from build123d import *

# Parameters (mm, degrees)
BOSS_EXTRUDE1_DEPTH  = 30
SHELL1_T             = -2
BOSS_EXTRUDE8_START  = -28
SKETCH10_R           = 1.25
BOSS_EXTRUDE8_DEPTH  = 28
BOSS_EXTRUDE10_START = 10
SKETCH4_R            = 2.7
BOSS_EXTRUDE10_DEPTH = 2.7
LPATTERN1_COUNT      = 4
LPATTERN1_PITCH      = 25
SKETCH15_R           = 2.7
BOSS_EXTRUDE11_DEPTH = 2.7


with BuildPart() as part:
    # Sketch3 → Boss-Extrude1 (new body)
    with BuildSketch(Plane.XY):
        Polygon((-5, -5), (105, -5), (105, 10), (143.418246447, 42.000599056), (124.217887014, 65.051546924), (107.928964784, 51.483637987), (105, 55), (105, 100), (-5, 100), align=None)
    extrude(amount=BOSS_EXTRUDE1_DEPTH)

    # Shell1
    shell1_openings = [part.faces().sort_by_distance(p)[0] for p in [
        (56.242959197, 46.819948693, 30),
    ]]
    offset(amount=SHELL1_T, openings=shell1_openings, kind=Kind.INTERSECTION)

    # Sketch10 → Boss-Extrude8 (add)
    # profile 1 of 4: a face of its own
    with BuildSketch(Plane.XY.offset(30).offset(BOSS_EXTRUDE8_START)):
        with BuildLine():
            Line((98, 98), (103, 98))
            Line((103, 98), (103, 93))
            ThreePointArc((103, 93), (99.464466094, 94.464466094), (98, 98))
        make_face()
        with Locations(Location((101.232233047, 96.232233047, 0), (0, 0, 180))):
            Circle(SKETCH10_R, mode=Mode.SUBTRACT)
    # profile 2 of 4: a face of its own
    with BuildSketch(Plane.XY.offset(30).offset(BOSS_EXTRUDE8_START)):
        with BuildLine():
            Line((103, 2), (103, -3))
            Line((103, -3), (98, -3))
            ThreePointArc((98, -3), (99.464466094, 0.535533906), (103, 2))
        make_face()
        with Locations(Location((101.232233047, -1.232233047, 0), (0, 0, 180))):
            Circle(SKETCH10_R, mode=Mode.SUBTRACT)
    # profile 3 of 4: a face of its own
    with BuildSketch(Plane.XY.offset(30).offset(BOSS_EXTRUDE8_START)):
        with BuildLine():
            Line((-3, 2), (-3, -3))
            Line((-3, -3), (2, -3))
            ThreePointArc((2, -3), (0.535533906, 0.535533906), (-3, 2))
        make_face()
        with Locations(Location((-1.232233047, -1.232233047, 0), (0, 0, 180))):
            Circle(SKETCH10_R, mode=Mode.SUBTRACT)
    # profile 4 of 4: a face of its own
    with BuildSketch(Plane.XY.offset(30).offset(BOSS_EXTRUDE8_START)):
        Polygon((103, 54.276153954), (103, 44.775111449), (107.672258888, 48.666884167), align=None)
        with Locations(Location((104.838291581, 48.944255676, 0), (0, 0, 180))):
            Circle(SKETCH10_R, mode=Mode.SUBTRACT)
    extrude(amount=BOSS_EXTRUDE8_DEPTH)

    # Sketch4 → Boss-Extrude10 (add)
    with BuildSketch(Plane(origin=(0, 0, 0), x_dir=(0, 0, -1), z_dir=(1, 0, 0)).offset(BOSS_EXTRUDE10_START)):
        with BuildLine():
            Line((-25, 100), (-13, 100))
            Line((-13, 100), (-13, 106))
            ThreePointArc((-13, 106), (-19, 112), (-25, 106))
            Line((-25, 106), (-25, 100))
        make_face()
        with Locations(Location((-19, 106, 0), (0, 0, 180))):
            Circle(SKETCH4_R, mode=Mode.SUBTRACT)
    boss_extrude10 = extrude(amount=BOSS_EXTRUDE10_DEPTH)

    # LPattern1: Boss-Extrude10 ×4
    with Locations(*[(i * LPATTERN1_PITCH, 0, 0) for i in range(1, LPATTERN1_COUNT)]):
        add(boss_extrude10)

    # Sketch15 → Boss-Extrude11 (add)
    with BuildSketch(Plane(origin=(28.491802957, -34.205769267, 0), x_dir=(-0.7683649289406903, -0.6400119811175163, 0), z_dir=(0.6400119811175163, -0.7683649289406903, 0))):
        with BuildLine():
            Line((-137.07843735, -13), (-143.07843735, -13))
            ThreePointArc((-143.07843735, -13), (-149.07843735, -19), (-143.07843735, -25))
            Line((-143.07843735, -25), (-137.07843735, -25))
            Line((-137.07843735, -25), (-137.07843735, -13))
        make_face()
        with Locations(Location((-143.07843735, -19, 0), (0, 0, 180))):
            Circle(SKETCH15_R, mode=Mode.SUBTRACT)
    extrude(amount=BOSS_EXTRUDE11_DEPTH)


solid = part.part
Build history of the part. All positions in model axes, mm. A direction names the side the tool comes from. Round coordinates to 2 decimals unless told otherwise and drop trailing zeros. Order: outer loops, then holes, each group sorted by start corner. A loop starts at its lowest first (then second) coordinate and runs counter-clockwise, first axis right, second up. Notation, with made-up numbers: M 74.25,79.25 L 127.25,79.25 A7 cw 127.25,88.25 Z; hole C 29.25,-37.5 d9. An arc over 180 degrees is marked long. Use CSV: the item, a comma, the result in double quotes. Start each with the question number.
(1) Cut at D-D on z = 19. State how many separate pieces and enclosed holes the cut face has, then the cut area to 3 significant figures.
(2) Drill centre lines: probe 1 along Y at (x, z) = (36.5, 19); probe 2 along Y at (x, z) = (93, 20.5); probe 3 along X at (y, z) = (8.5, 4.75). Where is each one in solid material? Low to high.
(3) Cut at B-B on x = 96. List the corners of the cut face in (y, z), then the cut area to 3 significant figures.
(4) Flat gauge pins, fed straight in: P1, Ø3.5, axis at y = 108, z = 16.5, coming from the +X side; P2, Ø3, axis at x = 11.5, y = 103, coming from the +Z side; P3, Ø13, axis at y = 106, z = 21.5, coming from the +X side. Where does each tip first touch, or does it go through?
(5) Mould opens along Y. For faces 1 (the face through (10, 103, 18)), 2 (the face through (106.5, 53.2, 14.8)), 3 (the face through (138.172, 53.639, 20.249)) say: +Y half, -Y half, draft (parallel to the pull), parting line (faces both ways), or undercut.
(6) Tool access for faces 4 (the face through (-5, 48, 15)), 5 (the face through (137, 54, 25)), 6 (the face through (87.7, 103, 18)), 7 (the face through (99, 0, 16)), 8 (the face through (116.187, 58.363, 14.79)): list every direction of +Z, -Z, +X, -X, +Y, -Y with a clear straight run to the whole face (end or side of a thin tool).
(7) Cut at C-C on z = 5.5. List the corners of the cut face in (x, y).
(8) Cut at A-A on y = 4.5. List the corners of the cut face in (x, z), then the cut area to 3 significant figures.
Findings:
1,separate pieces,"6"
1,enclosed holes,"5"
1,area,"1,120 mm^2"
2,probe 1,"y = -5 to -3, 98 to 103.3, 108.7 to 112"
2,probe 2,"y = -5 to -3, 98 to 100"
2,probe 3,"x = -5 to -3, 103 to 105"
3,outline,"M -5,0 L 100,0 L 100,30 L 98,30 L 98,2 L -3,2 L -3,30 L -5,30 Z"
3,area,"322 mm^2"
4,P1,"stops at x = 87.7"
4,P2,"stops at z = 25"
4,P3,"stops at x = 105"
5,face 1,"draft"
5,face 2,"+Y half"
5,face 3,"undercut"
6,face 4,"+Z, -Z, -X, +Y, -Y"
6,face 5,"+Z, +X, +Y"
6,face 6,"+Z, -Z, +X, +Y"
6,face 7,"+Z"
6,face 8,"+Z, -Z, +Y"
7,outline,"M -5,-5 L 105,-5 L 105,10 L 143.42,42 L 124.22,65.05 L 107.93,51.48 L 105,55 L 105,100 L -5,100 Z; hole M -3,2 A5 cw 2,-3 L 98,-3 A5 cw 103,2 L 103,10.94 L 140.6,42.26 L 123.96,62.23 L 103,44.78 L 103,93 A5 cw 98,98 L -3,98 Z; hole C -1.23,-1.23 d2.5; hole C 101.23,-1.23 d2.5; hole C 101.23,96.23 d2.5; hole C 104.84,48.94 d2.5"
8,outline,"M -5,0 L 105,0 L 105,30 L 103,30 L 103,2 L -3,2 L -3,30 L -5,30 Z"
8,area,"332 mm^2"
